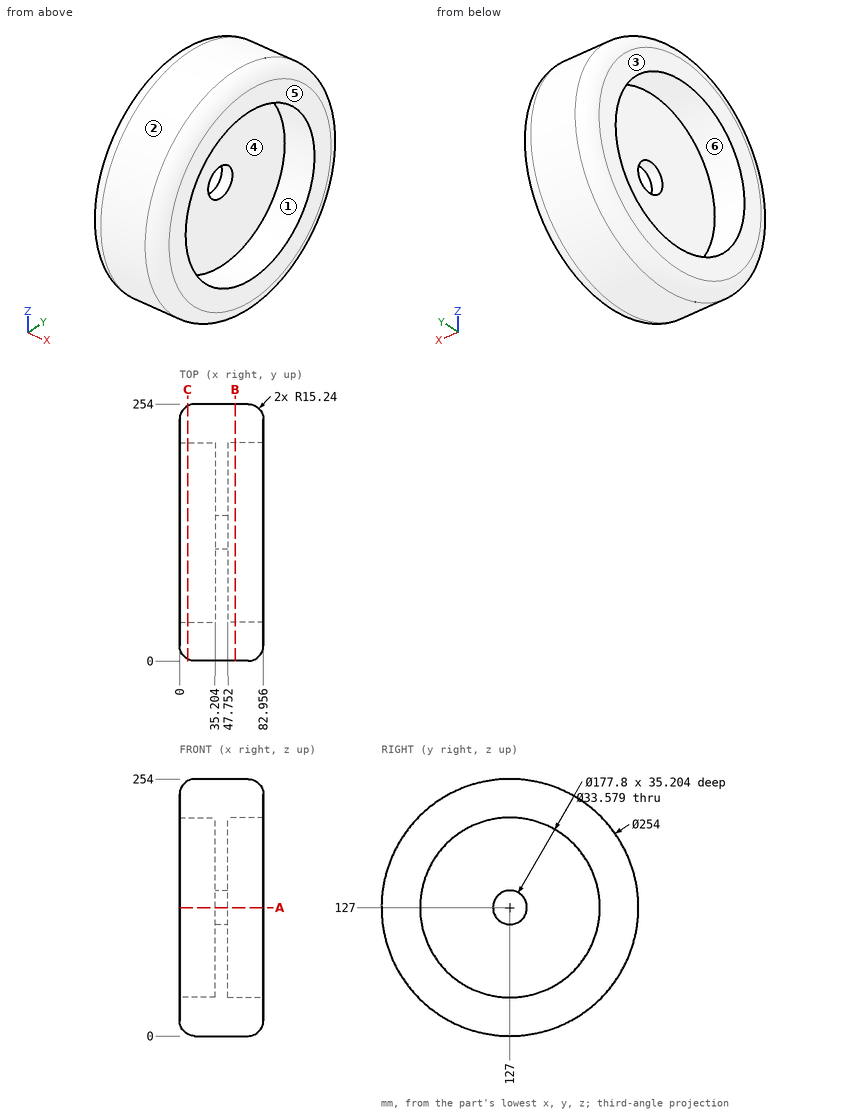
Job drawing, mm, ordinate dimensions from the low corner. One solid piece. A direction names the side the tool comes from. Give positions to 0.01 mm unless a question says otherwise; leave off trailing zeros. Loops run counter-clockwise (first coordinate to the right, second up) from the corner with the lowest first, then second, coordinate; pieces in that order, holes last.
Item 1: Slice it at B-B, the plane x = 55. List the corners of the cut face in (y, z).
Answers follow:
outline: circle Ø254 at (127, 127); hole circle Ø177.8 at (127, 127)
Item 2: Slice it at C-C, the plane x = 8. List the corners of the cut face in (y, z), and give its area (3 significant figures).
Answers follow:
outline: circle Ø250.34 at (127, 127); hole circle Ø177.8 at (127, 127)
area: 24,400 mm2
Item 3: Slice it at A-A, the plane z = 127. List the corners of the cut face in (x, y) (1 decimal), and give its area (3 significant figures).
Answers follow:
outline: (0, 15.2) arc R15.2 ccw to (15.2, 0) - (67.7, 0) arc R15.2 ccw to (83, 15.2) - (83, 38.1) - (47.8, 38.1) - (47.8, 110.2) - (35.2, 110.2) - (35.2, 38.1) - (0, 38.1) - close; (0, 215.9) - (35.2, 215.9) - (35.2, 143.8) - (47.8, 143.8) - (47.8, 215.9) - (83, 215.9) - (83, 238.8) arc R15.2 ccw to (67.7, 254) - (15.2, 254) arc R15.2 ccw to (0, 238.8) - close
area: 7,930 mm2
Item 4: Pull direction Z, two halves, no side cores. Call the marked faces 1, 2, 3 and 4: released by +Z, released by -Z, zero draft, split by the parting line, or undercut.
Answers follow:
face 1: undercut
face 2: split by the parting line
face 3: zero draft
face 4: undercut
Item 5: Drill centre lines: line 1 (Z direction, x = 61, y = 166.5); line 2 (X direction, y = 141, z = 207.5) (1 decimal); line 3 (Z direction, x = 62, y = 186.5). Where is each one in solid material? Low to high.
Answers follow:
line 1: z = 6.3 to 47.36, 206.64 to 247.7
line 2: x = 35.2 to 47.8
line 3: z = 14.8 to 60.95, 193.05 to 239.2
Item 6: Flat gauge pins, fed straight in: pin 1 (12 mm diameter, centred on y = 118.5, z = 190.5, fed in from -X); pin 2 (5 mm diameter, centred on x = 40, y = 187, fed in from -Z); pin 3 (5 mm diameter, centred on x = 58.5, z = 110.5, fed in from -Y); pin 4 (4 mm diameter, centred on y = 221.5, z = 136, fed in from -X). Where does each tip first touch, or does it go through?
Answers follow:
pin 1: stops at x = 35.2
pin 2: stops at z = 13.76
pin 3: stops at y = 0.77
pin 4: stops at x = 0
Item 7: Which spindle directions (+Z, -Z, +X, -X, +Y, -Y) get a long thin tool onto all of the face, cutting with end or side? Do the marked faces 5 and 6. Say none if no direction does.
Answers follow:
face 5: +Z, -Z, +X, +Y, -Y
face 6: -X
